from build123d import *

# Parameters (mm, degrees)
F0_W     = 52.3875
F0_H     = 52.3875
F0_W_2   = 39.6875
F0_H_2   = 39.6875
F1_DEPTH = 19.05
F2_R     = 1.5875
F3_DEPTH = 25.4
F2_R_2   = 4.7625
F4_DEPTH = 3.175
F6_D     = 3.175


with BuildPart() as f1:
    # F0 (on Top) → F1 (new body)
    with BuildSketch(Plane.XY):
        with Locations((19.05, 19.05)):
            Rectangle(F0_W, F0_H)
        with Locations((19.05, 19.05)):
            Rectangle(F0_W_2, F0_H_2, mode=Mode.SUBTRACT)
    extrude(amount=F1_DEPTH)

    # F2 (on face) → F3 (cut)
    with BuildSketch(Plane.XZ.offset(-38.89375)):
        with Locations((19.05, 9.525)):
            Circle(F2_R)
    extrude(amount=-F3_DEPTH, mode=Mode.SUBTRACT)

    # F2 (on face) → F4 (cut)
    with BuildSketch(Plane.XZ.offset(-38.89375)):
        with Locations((19.05, 9.525)):
            Circle(F2_R_2)
        with Locations((19.05, 9.525)):
            Circle(F2_R, mode=Mode.SUBTRACT)
    extrude(amount=-F4_DEPTH, mode=Mode.SUBTRACT)

    # F6 (through all)
    with Locations(Plane.XZ.offset(7.14375)):
        with Locations((19.05, 9.525)):
            Hole(F6_D / 2)


solid = f1.part
Work out the finished part from the listing and answer in its coordinate system (mm). A direction names the side the tool comes from. Give positions to 0.01 mm unless a question says otherwise; leave off trailing zeros. Loops run counter-clockwise (first coordinate to the right, second up) from the corner with the lowest first, then second, coordinate; pieces in that order, holes last. Notation, with made-up numbers: M 87.5,10.5 L 94.5,10.5 A21 cw 94.5,27.5 Z; hole C -0.5,-1 d6. An arc over 180 degrees is marked long. Use CSV: the item, a comma, the result in double quotes.
1) Find section D-D on z = 7.25. Write down the section's boundary in (x, y), plus the area to 3 significant figures.
Answer:
outline,"M -7.14,-7.14 L 45.24,-7.14 L 45.24,45.24 L -7.14,45.24 Z; hole M -0.79,-0.79 L 38.89,-0.79 L 38.89,38.89 L 23.23,38.89 L 23.23,42.07 L 14.87,42.07 L 14.87,38.89 L -0.79,38.89 Z"
area,"1,140 mm^2"
2) Determine the mould class of faces 1 (the flat face through (19, -7.144, 12)), 2 (the flat face through (-7.144, 19, 9)), 3 (the flat face through (14, 38.894, 12)), 4 (the flat face through (19, 45.244, 12)) for opening direction Y: released by +Y, released by -Y, zero draft, split by the parting line, or undercut.
Answer:
face 1,"released by -Y"
face 2,"zero draft"
face 3,"undercut"
face 4,"released by +Y"
3) Consider L1, parallel to X at y = 29, z = 12.5; L2, parallel to Y at x = 17.5, z = 10.5. Determine where each line is inside the solid, lowest interval first.
Answer:
L1,"-7.14 to -0.79, 38.89 to 45.24"
L2,"-7.14 to -0.79, 42.07 to 45.24"
4) Which of the six approach directions +Z, -Z, +X, -X, +Y, -Y give full straight-line access (tool end or side, diameter ignored) to faces 5 (the cylindrical face through (19.394, -3.924, 7.975)), 6 (the flat face through (18, 42.069, 11)), 7 (the flat face through (-0.794, 19, 9))?
Answer:
face 5,"+Y, -Y"
face 6,"none"
face 7,"+Z, -Z"
5) Find section A-A on x = 19.05. Write down the section's boundary in (y, z).
Answer:
outline,"M -7.14,0 L -0.79,0 L -0.79,7.94 L -7.14,7.94 Z; M -7.14,11.11 L -0.79,11.11 L -0.79,19.05 L -7.14,19.05 Z; M 38.89,0 L 45.24,0 L 45.24,7.94 L 42.07,7.94 L 42.07,4.76 L 38.89,4.76 Z; M 38.89,14.29 L 42.07,14.29 L 42.07,11.11 L 45.24,11.11 L 45.24,19.05 L 38.89,19.05 Z"
6) Find section B-B on y = 9. Write down the section's boundary in (x, z), plus the area to 3 significant figures.
Answer:
outline,"M -7.14,0 L -0.79,0 L -0.79,19.05 L -7.14,19.05 Z; M 38.89,0 L 45.24,0 L 45.24,19.05 L 38.89,19.05 Z"
area,"242 mm^2"
